from build123d import *

# Parameters (mm, degrees)
SKETCH_W        = 10
SKETCH_H        = 10
PAD_DEPTH       = 4.5
SKETCH001_R     = 2.05
POCKET_DEPTH    = 2
SKETCH006_W     = 6
SKETCH006_H     = 8
SKETCH006_W_2   = 2.5
SKETCH006_H_2   = 2.5
POCKET003_DEPTH = 0.1
SKETCH007_R     = 0.5
POCKET004_DEPTH = 0.1
SKETCH008_W     = 1
SKETCH008_H     = 1
POCKET005_DEPTH = 1


with BuildPart() as part:
    # Sketch → Pad (new body)
    with BuildSketch(Plane.XY):
        with Locations((5, 5)):
            Rectangle(SKETCH_W, SKETCH_H)
    extrude(amount=PAD_DEPTH)

    # Sketch001 (on Face6 of Pad) → Pocket (cut)
    with BuildSketch(Plane.XY.offset(4.5)):
        with Locations((5, 5)):
            Circle(SKETCH001_R)
    extrude(amount=-POCKET_DEPTH, mode=Mode.SUBTRACT)

    # Sketch006 → Pocket003 (cut)
    with BuildSketch(Plane.XY):
        with Locations((5, 5)):
            Rectangle(SKETCH006_W, SKETCH006_H)
        with Locations((5, 5)):
            Rectangle(SKETCH006_W_2, SKETCH006_H_2, mode=Mode.SUBTRACT)
    extrude(amount=POCKET003_DEPTH, mode=Mode.SUBTRACT)

    # Sketch007 → Pocket004 (cut)
    with BuildSketch(Plane.XY):
        with Locations((5, 5)):
            Circle(SKETCH007_R)
    extrude(amount=POCKET004_DEPTH, mode=Mode.SUBTRACT)

    # Sketch008 → Pocket005 (cut)
    with BuildSketch(Plane.XY):
        with Locations((0.5, 7.54)):
            Rectangle(SKETCH008_W, SKETCH008_H)
        with Locations((0.5, 5)):
            Rectangle(SKETCH008_W, SKETCH008_H)
        with Locations((0.5, 2.46)):
            Rectangle(SKETCH008_W, SKETCH008_H)
        with Locations((9.5, 7.54)):
            Rectangle(SKETCH008_W, SKETCH008_H)
        with Locations((9.5, 5)):
            Rectangle(SKETCH008_W, SKETCH008_H)
        with Locations((9.5, 2.46)):
            Rectangle(SKETCH008_W, SKETCH008_H)
    extrude(amount=POCKET005_DEPTH, mode=Mode.SUBTRACT)


solid = part.part
Input: part model. Units: mm. Frame: model coordinates. A direction names the side the tool comes from. Coordinates: 2 decimals unless noted, no trailing zeros. Loops run counter-clockwise (first coordinate to the right, second up) from the corner with the lowest first, then second, coordinate; pieces in that order, holes last. Notation, with made-up numbers: (73.5, -30) - (127.5, -30) arc R24 ccw to (127.5, 3) - close; hole circle Ø7 at (12, 2). An arc over 180 degrees is marked (long way). Answer in a Markdown table with one row per item. Add a question column.
Item 1: Contact query for flat-ended pins moving along their axis: P1, Ø0.8, axis at x = 9.5, y = 5, coming from the -Z side; P2, Ø0.8, axis at x = 5, y = 5, coming from the -Z side; P3, Ø0.5, axis at y = 2.5, z = 0.5, coming from the +X side. Output: stop coordinate, or through.
Item 2: Access query for faces 4 (the flat face through (0.5, 2.5, 1)), 5 (the flat face through (9.5, 5, 1)), 6 (the flat face through (5, 5, 0.1)), 7 (the flat face through (5, 5, 2.5)). Directions: +Z, -Z, +X, -X, +Y, -Y. A direction counts if a zero-diameter tool reaches every point of the face in a straight line with its end or side. Return the directions, or none.
Item 3: Section query C-C on x = 9.25. Return the cut outline in (y, z).
Item 4: Section query D-D on x = 2.75. Return the cut outline in (y, z), then the cut area to 3 significant figures.
Item 5: Section query A-A on z = 3.4. Return the cut outline in (x, y), then the cut area to 3 significant figures.
Item 6: Section query B-B on y = 5. Return the cut outline in (x, z), then the cut area to 4 significant figures.
Item 7: Mould query, pull axis Y, two halves, no side actions, for faces 1 (the flat face through (9.5, 4.5, 0.5)), 2 (the flat face through (5, 10, 2)), 3 (the flat face through (1.6, 5.1, 0)). Classes: released by +Y, released by -Y, zero draft, split by the parting line, or undercut.
Item 8: Line query: line 1 along Y through (x, z) = (5, 3.55); line 2 along Z through (x, y) = (6.5, 6); line 3 along Y through (x, z) = (6, 2.6). Output: solid intervals per line, ascending. Write a range as [from, to].
Recorded:
| question | item | result |
|---|---|---|
| 1 | P1 | z = 1 |
| 1 | P2 | z = 0.1 |
| 1 | P3 | x = 9 |
| 2 | face 4 | -Z, -X |
| 2 | face 5 | -Z, +X |
| 2 | face 6 | -Z |
| 2 | face 7 | +Z |
| 3 | outline | (0, 0) - (1.96, 0) - (1.96, 1) - (2.96, 1) - (2.96, 0) - (4.5, 0) - (4.5, 1) - (5.5, 1) - (5.5, 0) - (7.04, 0) - (7.04, 1) - (8.04, 1) - (8.04, 0) - (10, 0) - (10, 4.5) - (0, 4.5) - close |
| 4 | outline | (0, 0) - (1, 0) - (1, 0.1) - (9, 0.1) - (9, 0) - (10, 0) - (10, 4.5) - (0, 4.5) - close |
| 4 | area | 44.2 mm^2 |
| 5 | outline | (0, 0) - (10, 0) - (10, 10) - (0, 10) - close; hole circle Ø4.1 at (5, 5) |
| 5 | area | 86.8 mm^2 |
| 6 | outline | (0, 1) - (1, 1) - (1, 0) - (2, 0) - (2, 0.1) - (3.75, 0.1) - (3.75, 0) - (4.5, 0) - (4.5, 0.1) - (5.5, 0.1) - (5.5, 0) - (6.25, 0) - (6.25, 0.1) - (8, 0.1) - (8, 0) - (9, 0) - (9, 1) - (10, 1) - (10, 4.5) - (7.05, 4.5) - (7.05, 2.5) - (2.95, 2.5) - (2.95, 4.5) - (0, 4.5) - close |
| 6 | area | 34.35 mm^2 |
| 7 | face 1 | undercut |
| 7 | face 2 | released by +Y |
| 7 | face 3 | zero draft |
| 8 | line 1 | [0, 2.95], [7.05, 10] |
| 8 | line 2 | [0.1, 2.5] |
| 8 | line 3 | [0, 3.21], [6.79, 10] |
